from build123d import *

# Parameters (mm, degrees)
SKETCH_W     = 136
SKETCH_H     = 44
SKETCH_R     = 1.25
PAD_DEPTH    = 3
SKETCH001_W  = 44
SKETCH001_H  = 5
POCKET_DEPTH = 3.001
FILLET_R     = 2


with BuildPart() as part:
    # Sketch → Pad (new body)
    with BuildSketch(Plane.XZ):
        with Locations((68, 22)):
            Rectangle(SKETCH_W, SKETCH_H)
        with Locations((5, 22)):
            Circle(SKETCH_R, mode=Mode.SUBTRACT)
        with Locations((131, 22)):
            Circle(SKETCH_R, mode=Mode.SUBTRACT)
    extrude(amount=PAD_DEPTH)

    # Sketch001 (on Face8 of Pad) → Pocket (cut, through all)
    with BuildSketch(Plane.XZ.offset(3)):
        with Locations((70.7, 42.5)):
            Rectangle(SKETCH001_W, SKETCH001_H)
    extrude(amount=-POCKET_DEPTH, mode=Mode.SUBTRACT)

    # Fillet
    fillet_edges = [part.edges().sort_by_distance(p)[0] for p in [
        (48.7, -1.5, 40),
        (92.7, -1.5, 40),
    ]]
    fillet(fillet_edges, radius=FILLET_R)


solid = part.part
The model under review builds one solid part; all positions refer to its coordinate system, in mm. Round coordinates to 2 decimals unless told otherwise and drop trailing zeros. Order: outer loops, then holes, each group sorted by start corner. A loop starts at its lowest first (then second) coordinate and runs counter-clockwise, first axis right, second up. Notation, with made-up numbers: (82, 55) -> (122, 55) arc R21 ccw to (122, 83) -> close; hole circle Ø10 at (72, 74). An arc over 180 degrees is marked (long way). Return JSON: item names as keys, results as strings.
1. Take a section at B-B (x = 131). Write out the cut boundary in (y, z).
Answer block:
{"outline": "(-3, 0) -> (0, 0) -> (0, 20.75) -> (-3, 20.75) -> close; (-3, 23.25) -> (0, 23.25) -> (0, 44) -> (-3, 44) -> close"}
2. Take a section at A-A (z = 22). Write out the cut boundary in (x, y).
Answer block:
{"outline": "(0, -3) -> (3.75, -3) -> (3.75, 0) -> (0, 0) -> close; (6.25, -3) -> (129.75, -3) -> (129.75, 0) -> (6.25, 0) -> close; (132.25, -3) -> (136, -3) -> (136, 0) -> (132.25, 0) -> close"}
3. For L1, parallel to Z at x = 131, y = -2; L2, parallel to Z at x = 82, y = -2.35, list the stretches that pass through material, from the lowest coordinate up. Write a range as [from, to].
Answer block:
{"L1": "z = [0, 20.75], [23.25, 44]", "L2": "z = [0, 40]"}
4. Take a section at D-D (x = 60.5). Write out the cut boundary in (y, z), then the cut area to 3 significant figures.
Answer block:
{"outline": "(-3, 0) -> (0, 0) -> (0, 40) -> (-3, 40) -> close", "area": "120 mm²"}
5. Insertion check: P1, Ø3, axis at x = 5, z = 22, coming from the -Y side. The pin has a flat end and moves straight along its axis. Give the tip position at first contact, or say it passes through.
Answer block:
{"P1": "stops at y = -3"}
6. Take a section at C-C (y = -2.05). Write out the cut boundary in (x, z), then the cut area to 3 significant figures.
Answer block:
{"outline": "(0, 0) -> (136, 0) -> (136, 44) -> (92.7, 44) -> (92.7, 42) arc R2 cw to (90.7, 40) -> (50.7, 40) arc R2 cw to (48.7, 42) -> (48.7, 44) -> (0, 44) -> close; hole circle Ø2.5 at (5, 22); hole circle Ø2.5 at (131, 22)", "area": "5,800 mm²"}
7. The part is to be moulded in two halves that separate along X. For faces 1 (the face through (136, -1, 22)), 2 (the face through (70, -2, 40)), 3 (the face through (67, -3, 22)), say which applies: +X half, -X half, draft (parallel to the pull), parting line (faces both ways), or undercut.
Answer block:
{"face 1": "+X half", "face 2": "undercut", "face 3": "draft"}
